Check sheet for the modelled part. Datum: model origin and axes. Units: mm. Face numbers are marked on the shaded views. A direction names the side the tool comes from. Coordinates: 2 decimals unless noted, no trailing zeros. Write each loop counter-clockwise with the first axis right and the second up, starting at its lowest first coordinate (ties: lowest second). Pieces come first, ordered by that corner, then holes. Notation, with made-up numbers: (-39.5, -14) - (3.5, -14) arc R13 ccw to (3.5, 4) - close; hole circle Ø10 at (-39, 38). An arc over 180 degrees is marked (long way). Use one line per item in the form item = value. Start each with the question number.
1. Cross-section at A-A on x = 6. Record the boundary of the cut face in (y, z), then the cut area to 3 significant figures.
2. Draft check along X on the marked faces 1, 2 and 3. Enter one of: +X half, -X half, draft (parallel to the pull), parting line (faces both ways), or undercut.
3. Cross-section at D-D on z = -3.5. Record the boundary of the cut face in (x, y), then the cut area to 3 significant figures.
4. Tool access check on the marked faces 4 and 5. Record the directions out of +Z, -Z, +X, -X, +Y, -Y that give a thin tool (end or side, any length) a straight path to the whole face; none if there is none.
5. Cross-section at B-B on z = 6. Record the boundary of the cut face in (x, y).
6. Scan lines: line 1 along Y through (x, z) = (4.5, 2.5); line 2 along X through (y, z) = (6.5, 4); line 3 along Z through (x, y) = (4.25, 11.75). Record each from-to range of solid material in increasing order.
7. Go/stop test with flat-tipped pins: pin 1 Ø8 at (x, z) = (6, -9) entering from +Y; pin 2 Ø0.5 at (y, z) = (1, -13.5) entering from +X; pin 3 Ø1.3 at (y, z) = (1, -9) entering from -X. Record where each tip stops, or that it passes through.
8. Cross-section at C-C on y = 6.6. Record the boundary of the cut face in (x, z).
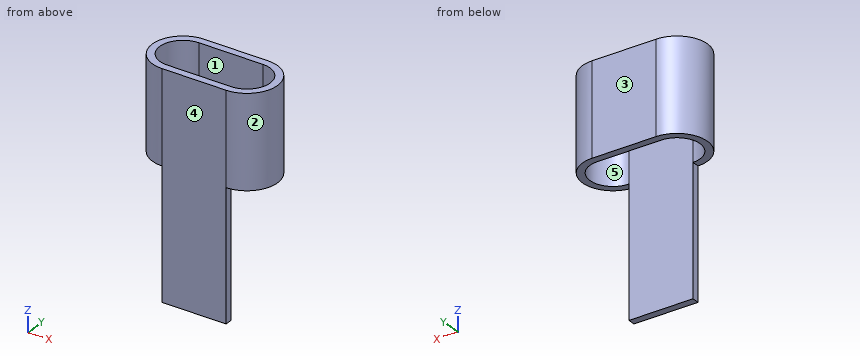
```python
from build123d import *

# Parameters (mm, degrees)
SKETCH1_W           = 14
SKETCH1_H           = 28
BOSS_EXTRUDE1_DEPTH = 1.6
SKETCH2_W           = 14
SKETCH2_H           = 1.6
BOSS_EXTRUDE2_DEPTH = 20


with BuildPart() as part:
    # Sketch1 → Boss-Extrude1 (new body)
    with BuildSketch(Plane(origin=(0, 0, 0), x_dir=(1, 0, 0), z_dir=(0, 1, 0))):
        with Locations((0, 14)):
            Rectangle(SKETCH1_W, SKETCH1_H)
    extrude(amount=BOSS_EXTRUDE1_DEPTH)

    # Sketch2 → Boss-Extrude2 (add)
    with BuildSketch(Plane.XY):
        with BuildLine():
            Line((-7, 13.2), (7, 13.2))
            ThreePointArc((7, 13.2), (13.6, 6.6), (7, 0))
            Line((7, 0), (7, 1.6))
            ThreePointArc((7, 1.6), (12, 6.6), (7, 11.6))
            Line((7, 11.6), (-7, 11.6))
            ThreePointArc((-7, 11.6), (-12, 6.6), (-7, 1.6))
            Line((-7, 1.6), (-7, 0))
            ThreePointArc((-7, 0), (-13.6, 6.6), (-7, 13.2))
        make_face()
        with Locations((0, 0.8)):
            Rectangle(SKETCH2_W, SKETCH2_H)
    extrude(amount=BOSS_EXTRUDE2_DEPTH)


solid = part.part
```
Final values:
q1.outline = (0, -28) - (1.6, -28) - (1.6, 20) - (0, 20) - close; (11.6, 0) - (13.2, 0) - (13.2, 20) - (11.6, 20) - close
q1.area = 109 mm²
q2.face_1 = undercut
q2.face_2 = +X half
q2.face_3 = draft
q3.outline = (-7, 0) - (7, 0) - (7, 1.6) - (-7, 1.6) - close
q3.area = 22.4 mm²
q4.face_4 = +Z, -Z, +X, -X, -Y
q4.face_5 = +Z, -Z
q5.outline = (-7, 0) - (7, 0) arc R6.6 ccw to (7, 13.2) - (-7, 13.2) arc R6.6 ccw to start; hole (-7, 1.6) - (7, 1.6) arc R5 ccw to (7, 11.6) - (-7, 11.6) arc R5 ccw to start
q6.line_1 = 0 to 1.6, 11.6 to 13.2
q6.line_2 = -13.6 to -12, 12 to 13.6
q6.line_3 = 0 to 20
q7.pin_1 = 1.6
q7.pin_2 = 7
q7.pin_3 = -7
q8.outline = (-13.6, 0) - (-12, 0) - (-12, 20) - (-13.6, 20) - close; (12, 0) - (13.6, 0) - (13.6, 20) - (12, 20) - close
